Design review of the part shown in the three views and the two pictorial views. Dimensions are in mm from the part's minimum x, y and z. Give positions to 0.01 mm unless a question says otherwise; leave off trailing zeros. Loops run counter-clockwise (first coordinate to the right, second up) from the corner with the lowest first, then second, coordinate; pieces in that order, holes last. Notation, with made-up numbers: M 13,25 L 41,25 A8 ccw 41,37 Z; hole C 3.5,27 d5. An arc over 180 degrees is marked long. Return JSON: item names as keys, results as strings. Group by question number.
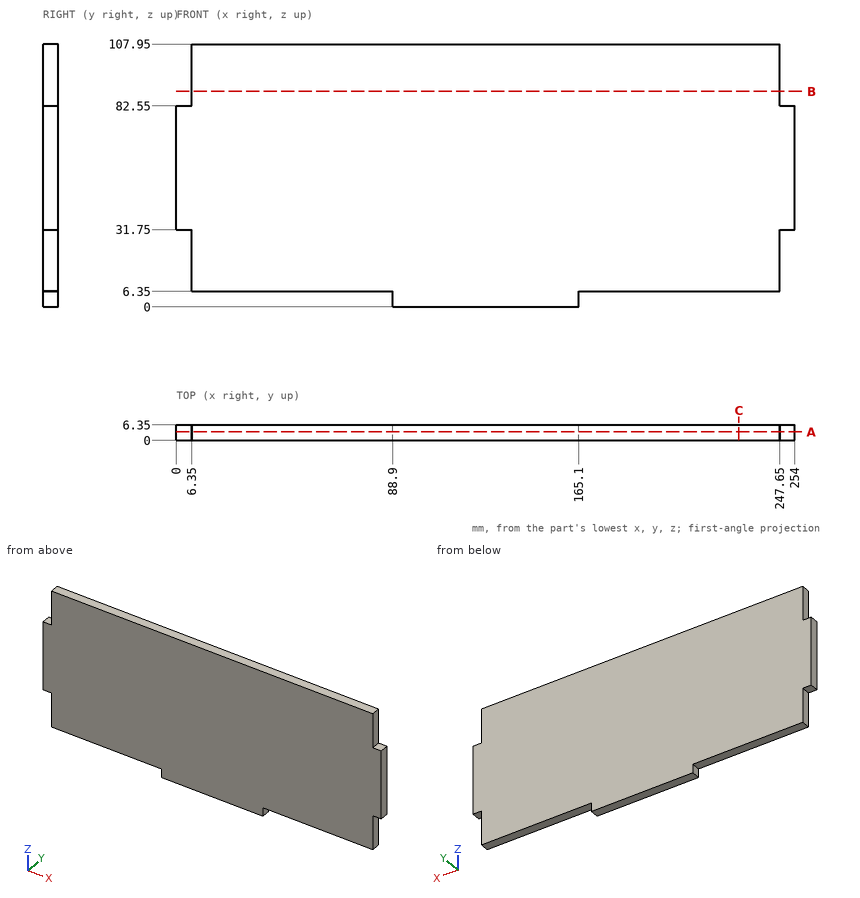
(1) Add section A-A (y = 3.5). Write out the cut boundary in (x, z), and give its area (3 significant figures).
(2) Add section B-B (z = 88.5). Write out the cut boundary in (x, y).
(3) For probe 1 along X at (y, z) = (1.5, 26); probe 2 along Z at (x, y) = (16, 5.25), list the stretches that pass through material, from the lowest coordinate up.
(4) Add section C-C (x = 231). Write out the cut boundary in (y, z), and give its area (3 significant figures).
(5) For pin 1 (1 mm diameter, centred on x = 66.5, y = 2.5, fed in from -Z); pin 2 (3 mm diameter, centred on x = 251, y = 3.5, fed in from +Z); pin 3 (1 mm diameter, centred on x = 101, y = 1.5, fed in from -Z); pin 4 (1.9 mm diameter, centred on y = 2, z = 25, fed in from +X), all flat-tipped, find the tip position at first contact; note any pin that passes through.
Verdict:
{
 "1": {"outline": "M 0,31.75 L 6.35,31.75 L 6.35,6.35 L 88.9,6.35 L 88.9,0 L 165.1,0 L 165.1,6.35 L 247.65,6.35 L 247.65,31.75 L 254,31.75 L 254,82.55 L 247.65,82.55 L 247.65,107.95 L 6.35,107.95 L 6.35,82.55 L 0,82.55 Z", "area": "25,600 mm²"},
 "2": {"outline": "M 6.35,0 L 247.65,0 L 247.65,6.35 L 6.35,6.35 Z"},
 "3": {"probe 1": "x = 6.35 to 247.65", "probe 2": "z = 6.35 to 107.95"},
 "4": {"outline": "M 0,6.35 L 6.35,6.35 L 6.35,107.95 L 0,107.95 Z", "area": "645 mm²"},
 "5": {"pin 1": "stops at z = 6.35", "pin 2": "stops at z = 82.55", "pin 3": "stops at z = 0", "pin 4": "stops at x = 247.65"}
}
